Can you work these out from the model? Positions are in its coordinate system, mm. A direction names the side the tool comes from. Round coordinates to 2 decimals unless told otherwise and drop trailing zeros. Order: outer loops, then holes, each group sorted by start corner. A loop starts at its lowest first (then second) coordinate and runs counter-clockwise, first axis right, second up. Notation, with made-up numbers: (70, 25.5) -> (126, 25.5) arc R27 ccw to (126, 56.5) -> close; hole circle Ø4 at (36.25, -9.5). An arc over 180 degrees is marked (long way). Use a Markdown table: item, result. Add a question column.
Q1. For faces 4 (the face through (58, -270, -43)), 5 (the face through (201.12, -567.01, 13.69)), 6 (the face through (139, -2, -21)), 7 (the face through (139, 0, -23)), 8 (the face through (153.47, -94.83, -63.41)), which set-ups out of +Z, -Z, +X, -X, +Y, -Y let a thin tool reach every point of the face, with its end or its side?
Q2. If we section it at A-A on x = 141: List the corners of the cut face in (y, z) for me, plus the area to 3 significant figures.
Q3. I need wall thicknesses on line 1 along X through (y, z) = (-322, -52); line 2 along X through (y, z) = (-100, -61); line 3 along X through (y, z) = (-170.5, -7.5). Which ranges of each line are inside material? Lowest first, please. Write a range as [from, to].
Q4. We'd pull the mould along X, two halves only. Please class faces 1 (the face through (29, -118, -43)), 2 (the face through (273.445, -567.014, 20.979)), 3 (the face through (139, -280, -57)): +X half, -X half, draft (parallel to the pull), parting line (faces both ways), or undercut.
Q5. I'm going to push flat-ended pins straight in: pin 1 Ø1.6 at (x, y) = (124, -567) entering from +Z; pin 2 Ø4 at (x, y) = (145, -317.5) entering from +Z; pin 3 Ø1.6 at (x, y) = (228.5, -567.5) entering from -Z; pin 4 Ø6 at (x, z) = (199.5, 11.5) entering from +Y. Where does each tip first touch, or does it pass through?
Q6. If we section it at D-D on y = -460.5: List the corners of the cut face in (x, z) for me.
Q7. If we section it at C-C on z = -21.5: List the corners of the cut face in (x, y) for me, plus the area to 3 significant figures.
Q8. If we section it at B-B on y = -336: List the corners of the cut face in (x, z) for me.
```python
from build123d import *

# Parameters (mm, degrees)
F1_DEPTH  = 568
F3_DEPTH  = 2
F5_DEPTH  = 2
F6_R      = 12.5
F7_DEPTH  = 25
F8_R      = 13.5
F8_R_2    = 12.5
F9_DEPTH  = 13
F11_DEPTH = 25
F13_DEPTH = 25


with BuildPart() as f1:
    # F0 (on Front) → F1 (new body)
    with BuildSketch(Plane.XZ):
        Polygon((0, -55), (0, 0), (-2, 0), (-2, -57), (284, -57), (284, 0), (282, 0), (282, -55), align=None)
    extrude(amount=F1_DEPTH)

    # F2 (on Front) → F3 (join)
    with BuildSketch(Plane.XZ):
        with BuildLine():
            Line((0, 24), (0, 0))
            Line((0, 0), (0, -55))
            Line((0, -55), (282, -55))
            Line((282, -55), (282, 0))
            ThreePointArc((282, 0), (273.2132034356, 21.2132034356), (252, 30))
            Line((252, 30), (214, 30))
            ThreePointArc((214, 30), (211, 29.1961524227), (208.8038475773, 27))
            Line((208.8038475773, 27), (193.2153903092, 0))
            Line((193.2153903092, 0), (58.7846096908, 0))
            Line((58.7846096908, 0), (43.1961524227, 27))
            ThreePointArc((43.1961524227, 27), (41, 29.1961524227), (38, 30))
            Line((38, 30), (6, 30))
            ThreePointArc((6, 30), (1.7573593129, 28.2426406871), (0, 24))
        make_face()
        with BuildLine():
            ThreePointArc((17.5, 4), (13, 8.5), (17.5, 13))
            Line((17.5, 13), (23.5, 13))
            ThreePointArc((23.5, 13), (28, 8.5), (23.5, 4))
            Line((23.5, 4), (17.5, 4))
        make_face(mode=Mode.SUBTRACT)
        with BuildLine():
            ThreePointArc((225, 4), (220.5, 8.5), (225, 13))
            Line((225, 13), (235, 13))
            ThreePointArc((235, 13), (239.5, 8.5), (235, 4))
            Line((235, 4), (225, 4))
        make_face(mode=Mode.SUBTRACT)
    extrude(amount=F3_DEPTH)

    # F4 (on face) → F5 (join)
    with BuildSketch(Plane.XZ.offset(568)):
        with BuildLine():
            Line((0, 0), (0, -55))
            Line((0, -55), (282, -55))
            Line((282, -55), (282, 0))
            ThreePointArc((282, 0), (273.2132034356, 21.2132034356), (252, 30))
            Line((252, 30), (214, 30))
            ThreePointArc((214, 30), (211, 29.1961524227), (208.8038475773, 27))
            Line((208.8038475773, 27), (193.2153903092, 0))
            Line((193.2153903092, 0), (58.7846096908, 0))
            Line((58.7846096908, 0), (43.1961524227, 27))
            ThreePointArc((43.1961524227, 27), (41, 29.1961524227), (38, 30))
            Line((38, 30), (6, 30))
            ThreePointArc((6, 30), (1.7573593129, 28.2426406871), (0, 24))
            Line((0, 24), (0, 0))
        make_face()
        with BuildLine():
            ThreePointArc((17.5, 4), (13, 8.5), (17.5, 13))
            Line((17.5, 13), (23.5, 13))
            ThreePointArc((23.5, 13), (28, 8.5), (23.5, 4))
            Line((23.5, 4), (17.5, 4))
        make_face(mode=Mode.SUBTRACT)
        with BuildLine():
            ThreePointArc((225, 4), (220.5, 8.5), (225, 13))
            Line((225, 13), (235, 13))
            ThreePointArc((235, 13), (239.5, 8.5), (235, 4))
            Line((235, 4), (225, 4))
        make_face(mode=Mode.SUBTRACT)
    extrude(amount=-F5_DEPTH)

    # F6 (on face) → F7 (cut)
    with BuildSketch(Plane.XY.offset(-55)):
        with Locations((141, -100)):
            Circle(F6_R)
    extrude(amount=-F7_DEPTH, mode=Mode.SUBTRACT)

    # F8 (on face) → F9 (join)
    with BuildSketch(Plane(origin=(0, 0, -57), x_dir=(1, 0, 0), z_dir=(0, 0, -1))):
        with Locations((141, 100)):
            Circle(F8_R)
        with Locations((141, 100)):
            Circle(F8_R_2, mode=Mode.SUBTRACT)
    extrude(amount=F9_DEPTH)

    # F10 (on face) → F11 (join)
    with BuildSketch(Plane.XY.offset(-55)):
        with BuildLine():
            ThreePointArc((60, -120), (59.4142135624, -118.5857864376), (58, -118))
            Line((58, -118), (0, -118))
            Line((0, -118), (0, -120))
            Line((0, -120), (56, -120))
            ThreePointArc((56, -120), (57.4142135624, -120.5857864376), (58, -122))
            Line((58, -122), (58, -414))
            ThreePointArc((58, -414), (57.4142135624, -415.4142135624), (56, -416))
            Line((56, -416), (0, -416))
            Line((0, -416), (0, -418))
            Line((0, -418), (58, -418))
            ThreePointArc((58, -418), (59.4142135624, -417.4142135624), (60, -416))
            Line((60, -416), (60, -120))
        make_face()
    extrude(amount=F11_DEPTH)

    # F12 (on face) → F13 (cut)
    with BuildSketch(Plane.XY.offset(-55)):
        with BuildLine():
            Line((58, -414), (58, -122))
            ThreePointArc((58, -122), (57.4142135624, -120.5857864376), (56, -120))
            Line((56, -120), (0, -120))
            Line((0, -120), (0, -416))
            Line((0, -416), (56, -416))
            ThreePointArc((56, -416), (57.4142135624, -415.4142135624), (58, -414))
        make_face()
    extrude(amount=-F13_DEPTH, mode=Mode.SUBTRACT)


solid = f1.part
```
Answer below:
| question | item | result |
|---|---|---|
| 1 | face 4 | +Z, -Z |
| 1 | face 5 | +Z, +Y, -Y |
| 1 | face 6 | +Z |
| 1 | face 7 | +Z, -Z, +X, -X, +Y |
| 1 | face 8 | -Z |
| 2 | outline | (-568, -57) -> (-113.5, -57) -> (-113.5, -70) -> (-112.5, -70) -> (-112.5, -55) -> (-566, -55) -> (-566, 0) -> (-568, 0) -> close; (-87.5, -70) -> (-86.5, -70) -> (-86.5, -57) -> (0, -57) -> (0, 0) -> (-2, 0) -> (-2, -55) -> (-87.5, -55) -> close |
| 2 | area | 1,330 mm² |
| 3 | line 1 | [-2, 0], [58, 60], [282, 284] |
| 3 | line 2 | [127.5, 128.5], [153.5, 154.5] |
| 3 | line 3 | [-2, 0], [282, 284] |
| 4 | face 1 | undercut |
| 4 | face 2 | +X half |
| 4 | face 3 | draft |
| 5 | pin 1 | z = 0 |
| 5 | pin 2 | z = -55 |
| 5 | pin 3 | z = -57 |
| 5 | pin 4 | y = 0 |
| 6 | outline | (-2, -57) -> (284, -57) -> (284, 0) -> (282, 0) -> (282, -55) -> (0, -55) -> (0, 0) -> (-2, 0) -> close |
| 7 | outline | (-2, -568) -> (284, -568) -> (284, 0) -> (-2, 0) -> close; hole (0, -566) -> (282, -566) -> (282, -2) -> (0, -2) -> close |
| 7 | area | 3,400 mm² |
| 8 | outline | (-2, -57) -> (0, -57) -> (0, 0) -> (-2, 0) -> close; (58, -57) -> (284, -57) -> (284, 0) -> (282, 0) -> (282, -55) -> (60, -55) -> (60, -30) -> (58, -30) -> close |
